The listing builds one solid part. Answer for the finished solid, in the listing's coordinates (mm). A direction names the side the tool comes from. Coordinates: 2 decimals unless noted, no trailing zeros. Order: outer loops, then holes, each group sorted by start corner. A loop starts at its lowest first (then second) coordinate and runs counter-clockwise, first axis right, second up. Notation, with made-up numbers: (-38, -18.75) -> (-5, -18.75) arc R33 cw to (-5, 17.25) -> close; hole circle Ø11 at (-16.5, -19). An arc over 180 degrees is marked (long way). One line per question, with ' | ' between items.
Autodesk Inventor part; units mm, degrees
ref_plane "YZ Plane" through (0, 0, 0) normal (1, 0, 0) x (0, 1, 0)
ref_plane "XZ Plane" through (0, 0, 0) normal (0, 1, 0) x (-1, 0, 0)
ref_plane "XY Plane" through (0, 0, 0) normal (0, 0, 1) x (1, 0, 0)
sketch "Boceto1" plane through (0, 0, 0) normal (0, 0, 1) x (1, 0, 0)
  line L0 (0, 0) -> (60, 0)
  line L1 (60, 0) -> (60, 40)
  line L2 (60, 40) -> (0, 40)
  line L3 (0, 40) -> (0, 0)
  dimension "d0" = 60
  dimension "d1" = 40
extrude "Extrusión1" add sketch "Boceto1" along normal blind 40
sketch "Boceto2" plane through (0, 0, 40) normal (0, 0, 1) x (1, 0, 0)
  line L0 (0, 40) -> (0, 0)
  line L1 (0, 0) -> (5, 0)
  line L2 (0, 0) -> (0, 40)
  line L3 (0, 40) -> (5, 40)
  line L4 (5, 0) -> (5, 15)
  line L5 (0, 0) -> (60, 0)
  line L6 (5, 0) -> (20, 0) construction
  line L7 (5, 40) -> (5, 25)
  line L8 (60, 40) -> (0, 40)
  line L9 (5, 40) -> (20, 40) construction
  line L10 (5, 40) -> (25, 40) construction
  line L11 (25, 40) -> (25, 27.75) construction
  line L12 (25, 40) -> (37.25, 40) construction
  line L13 (5, 0) -> (25, 0) construction
  line L14 (25, 0) -> (25, 12.25) construction
  line L15 (5, 25) -> (25, 27.75)
  line L16 (5, 15) -> (25, 12.25)
  line L17 (25, 27.75) -> (25, 12.25)
  dimension "d4" = 5
  dimension "d5" = 40
  dimension "d6" = 5
  dimension "d7" = 15
  dimension "d8" = 90
  dimension "d9" = 15
  dimension "d10" = 90
  dimension "d11" = 20
  dimension "d12" = 12.25
  dimension "d13" = 90
  dimension "d14" = 20
  dimension "d15" = 12.25
  dimension "d16" = 90
extrude "Extrusión2" cut sketch "Boceto2" against normal blind 20
equation "\"d4\" = Espesor_corte"
equation "\"d6\" = Espesor_corte"
equation "\"Espesor_corte\" = 5"
equation "\"Angulo_0\" = 0"
equation "\"Angulo_90\" = 90deg"
properties part number "Hembra_parametrizada"
Item 1: Determine the mould class of faces 1 (the face through (30, 0, 20)), 2 (the face through (10, 20, 20)), 3 (the face through (5, 7, 30)), 4 (the face through (30, 40, 20)) for opening direction Y: pulls with the +Y half, pulls with the -Y half, needs draft (parallel to the pull), parting line crosses it, or undercut.
Computed values:
face 1: pulls with the -Y half | face 2: undercut | face 3: needs draft | face 4: pulls with the +Y half
Item 2: Find the intervals of material crossed by L1, parallel to Z at x = 15, y = 19.5; L2, parallel to X at y = 12, z = 28; L3, parallel to X at y = 20.5, z = 27, in increasing order.
Computed values:
L1: z = 0 to 20 | L2: x = 5 to 60 | L3: x = 25 to 60
Item 3: This flat-tipped pin is pushed along its axis until it touches: pin 1 Ø17 at (y, z) = (20.5, 29.5) entering from -X. Where does it stop, or does it pass through?
Computed values:
pin 1: stops at x = 5
Item 4: Section A-A, the plane z = 33 is taken. Give the vertices of the cut face in (x, y).
Computed values:
outline: (5, 0) -> (60, 0) -> (60, 40) -> (5, 40) -> (5, 25) -> (25, 27.75) -> (25, 12.25) -> (5, 15) -> close
Item 5: Section D-D, the plane y = 6 is taken. Give the vertices of the cut face in (x, z).
Computed values:
outline: (0, 0) -> (60, 0) -> (60, 40) -> (5, 40) -> (5, 20) -> (0, 20) -> close
Item 6: Section B-B, the plane y = 18 is taken. Give the vertices of the cut face in (x, z), plus the area to 3 significant figures.
Computed values:
outline: (0, 0) -> (60, 0) -> (60, 40) -> (25, 40) -> (25, 20) -> (0, 20) -> close | area: 1,900 mm^2
Item 7: Section C-C, the plane x = 15 is taken. Give the vertices of the cut face in (y, z) (3 decimals).
Computed values:
outline: (0, 0) -> (40, 0) -> (40, 40) -> (26.375, 40) -> (26.375, 20) -> (13.625, 20) -> (13.625, 40) -> (0, 40) -> close
Item 8: For faces 5 (the face through (25, 20, 30)), 6 (the face through (5, 33, 30)), 7 (the face through (30, 20, 0)), determine the directions among +Z, -Z, +X, -X, +Y, -Y from which every point of the face is accessible in a straight line to the end or side of a thin tool.
Computed values:
face 5: +Z | face 6: +Z, -X, +Y, -Y | face 7: -Z, +X, -X, +Y, -Y
